Input: part model. Units: mm. Frame: model coordinates. Round coordinates to 2 decimals unless told otherwise and drop trailing zeros. Loops run counter-clockwise (first coordinate to the right, second up) from the corner with the lowest first, then second, coordinate; pieces in that order, holes last. Notation, with made-up numbers: M -5.75,-7.75 L 15.25,-7.75 A28 ccw 15.25,26.25 Z; hole C 6,37.25 d9. An arc over 180 degrees is marked long. Return JSON: item names as keys, results as strings. Group by question number.
1) Section C-C (x = 34). Output: boundary loops of the cut face in (y, z).
2) Material intervals for line 1 (X direction, y = 0.6, z = 185); line 2 (Z direction, x = 142.4, y = 1.1); line 3 (X direction, y = 0.75, z = 117), sorted ascending. Write a range as from..to.
3) Section B-B (y = 2). Count the separate pieces of the cut face and the enclosed holes in it, plus the area to 3 significant figures.
4) Section A-A (z = 179). Output: boundary loops of the cut face in (x, y).
5) Section D-D (x = 119.5). Output: boundary loops of the cut face in (y, z), plus the area to 3 significant figures.
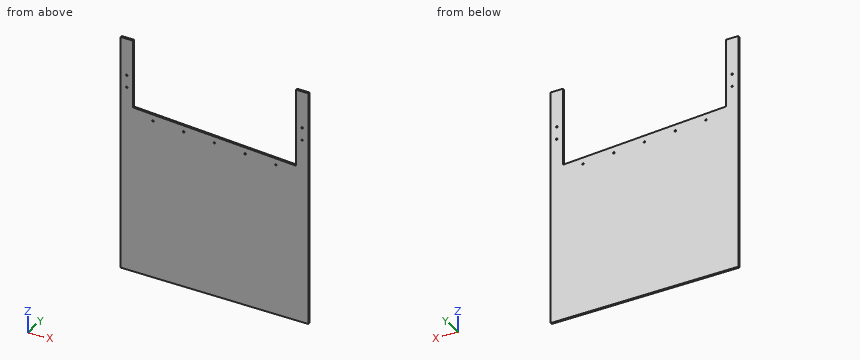
from build123d import *

# Parameters (mm, degrees)
BOSS_EXTRUDE1_DEPTH               = 3
BRUSH_HOLDER_MOUNTING_HOLES_D     = 2.5
BRUSH_HOLDER_MOUNTING_HOLES_DEPTH = 7.5
BRUSH_HOLDER_MOUNTING_HOLES_TIP   = 0.751075774
OMNI_BEARING_HOLES_D              = 2.5
OMNI_BEARING_HOLES_DEPTH          = 7.5
OMNI_BEARING_HOLES_TIP            = 0.751075774


with BuildPart() as part:
    # Sketch1 → Boss-Extrude1 (new body)
    with BuildSketch(Plane(origin=(0, 0, 0), x_dir=(1, 0, 0), z_dir=(0, 1, 0))):
        Polygon((-152.4, -135), (-152.4, -245), (-132.4, -245), (-132.4, -135), (132.4, -119.723076923), (132.4, -245), (152.4, -245), (152.4, -135), (152.4, 135), (-152.4, 135), align=None)
    extrude(amount=BOSS_EXTRUDE1_DEPTH)

    # Brush Holder Mounting Holes
    with Locations(Plane(origin=(0, 3, 0), x_dir=(1, 0, 0), z_dir=(0, 1, 0))):
        with Locations((0, -116.944245147), (-49.916997084, -119.824071902), (-99.833994168, -122.703898657), (49.916997084, -114.064418392), (99.833994168, -111.184591637)):
            Hole(BRUSH_HOLDER_MOUNTING_HOLES_D / 2, depth=BRUSH_HOLDER_MOUNTING_HOLES_DEPTH)
            with Locations((0, 0, -(BRUSH_HOLDER_MOUNTING_HOLES_DEPTH + BRUSH_HOLDER_MOUNTING_HOLES_TIP / 2))):  # 118° drill point
                Cone(0, BRUSH_HOLDER_MOUNTING_HOLES_D / 2, BRUSH_HOLDER_MOUNTING_HOLES_TIP, mode=Mode.SUBTRACT)

    # Omni-Bearing Holes
    with Locations(Plane(origin=(0, 0, 0), x_dir=(-1, 0, 0), z_dir=(0, -1, 0))):
        with Locations((-142.4, -165), (-142.4, -185), (142.4, -165), (142.4, -185)):
            Hole(OMNI_BEARING_HOLES_D / 2, depth=OMNI_BEARING_HOLES_DEPTH)
            with Locations((0, 0, -(OMNI_BEARING_HOLES_DEPTH + OMNI_BEARING_HOLES_TIP / 2))):  # 118° drill point
                Cone(0, OMNI_BEARING_HOLES_D / 2, OMNI_BEARING_HOLES_TIP, mode=Mode.SUBTRACT)


solid = part.part
Returned:
{
 "1": {"outline": "M 0,-135 L 3,-135 L 3,125.4 L 0,125.4 Z"},
 "2": {"line 1": "x = -152.4..-143.65, -141.15..-132.4, 132.4..141.15, 143.65..152.4", "line 2": "z = -135..163.75, 166.25..183.75, 186.25..245", "line 3": "x = -152.4..-1.25, 1.25..152.4"},
 "3": {"separate pieces": "1", "enclosed holes": "9", "area": "84,600 mm^2"},
 "4": {"outline": "M -152.4,0 L -132.4,0 L -132.4,3 L -152.4,3 Z; M 132.4,0 L 152.4,0 L 152.4,3 L 132.4,3 Z"},
 "5": {"outline": "M 0,-135 L 3,-135 L 3,120.47 L 0,120.47 Z", "area": "766 mm^2"}
}
